Autodesk Inventor part; units mm, degrees
ref_plane "YZ Plane" through (0, 0, 0) normal (1, 0, 0) x (0, 1, 0)
ref_plane "XZ Plane" through (0, 0, 0) normal (0, 1, 0) x (-1, 0, 0)
ref_plane "XY Plane" through (0, 0, 0) normal (0, 0, 1) x (1, 0, 0)
sketch "Sketch1" plane through (0, 0, 0) normal (1, 0, 0) x (0, 1, 0)
  circle A0 centre (0, 0) radius 18.5
  dimension "d0" = 37
extrude "Extrusion1" add sketch "Sketch1" along normal blind 27
sketch "Sketch2" plane through (0, 0, 0) normal (-1, 0, 0) x (0, 0, 1)
  circle A0 centre (0, 0) radius 16
  dimension "d3" = 32
extrude "Extrusion2" add sketch "Sketch2" along normal blind 34
sketch "Sketch3" plane through (27, 0, 0) normal (1, 0, 0) x (0, 0, -1)
  circle A0 centre (0, 15.5) radius 1.5
  circle A1 centre (-13.4234, 7.75) radius 1.5
  circle A2 centre (-13.4234, -7.75) radius 1.5
  circle A3 centre (0, -15.5) radius 1.5
  circle A4 centre (13.4234, -7.75) radius 1.5
  circle A5 centre (13.4234, 7.75) radius 1.5
  point P0 (0, 0)
  dimension "d8" = 3
  dimension "d9" = 15.5
  dimension "d12" = 360
extrude "Extrusion3" cut sketch "Sketch3" against normal blind 3
sketch "Sketch4" plane through (27, 0, 0) normal (1, 0, 0) x (0, 0, -1)
  circle A0 centre (-7, 0) radius 6
  point P0 (0, 0)
  dimension "d16" = 12
  dimension "d17" = 7
extrude "Extrusion4" add sketch "Sketch4" along normal blind 6
sketch "Sketch5" plane through (33, 0, 7) normal (1, 0, 0) x (0, 0, -1)
  circle A0 centre (0, 0) radius 3
  point P0 (7, 0)
  dimension "d20" = 6
  dimension "d21" = 7
extrude "Extrusion5" add sketch "Sketch5" along normal blind 15.5
properties part number "SPG30_Motor"
Input: part model. Units: mm. Frame: model coordinates. A direction names the side the tool comes from. Round coordinates to 2 decimals unless told otherwise and drop trailing zeros. Loops run counter-clockwise (first coordinate to the right, second up) from the corner with the lowest first, then second, coordinate; pieces in that order, holes last.
1) Pull-direction query (Y, two-part tool) for faces 3 (the cylindrical face through (25.52, -8.32, -14.81)), 4 (the flat face through (0, -6, 15)), 5 (the cylindrical face through (40.64, 1.15, 4.23)); classes: released by +Y, released by -Y, zero draft, split by the parting line, or undercut.
Ans:
face 3: undercut
face 4: zero draft
face 5: split by the parting line
2) Set-up query: faces 1 (the cylindrical face through (-16.76, 15.62, -3.47)), 2 (the cylindrical face through (25.521, -8.663, 14.614)). Return all of +Z, -Z, +X, -X, +Y, -Y with unobstructed straight access to the full face (end or side cutting, diameter ignored); none if empty.
Ans:
face 1: -X
face 2: +X
3) Section query B-B on y = 0. Return the cut outline in (x, z).
Ans:
outline: (-34, -16) - (0, -16) - (0, -18.5) - (27, -18.5) - (27, 1) - (33, 1) - (33, 4) - (48.5, 4) - (48.5, 10) - (33, 10) - (33, 13) - (27, 13) - (27, 18.5) - (0, 18.5) - (0, 16) - (-34, 16) - close
4) Section query A-A on z = 6. Return the cut outline in (x, y), plus the area to 3 significant figures.
Ans:
outline: (-34, -14.83) - (0, -14.83) - (0, -17.5) - (27, -17.5) - (27, -5.92) - (33, -5.92) - (33, -2.83) - (48.5, -2.83) - (48.5, 2.83) - (33, 2.83) - (33, 5.92) - (27, 5.92) - (27, 17.5) - (0, 17.5) - (0, 14.83) - (-34, 14.83) - close
area: 2,110 mm2
5) Pin query (flat end, axial travel): pin 1 (4 mm diameter, centred on x = 17.5, y = -2.5, fed in from -Z); pin 2 (10 mm diameter, centred on x = -24.5, y = 2.5, fed in from +Z); pin 3 (1.5 mm diameter, centred on y = -8, z = -13.5, fed in from +X). Return the tip coordinate at first contact, or that it passes through.
Ans:
pin 1: stops at z = -18.49
pin 2: stops at z = 16
pin 3: stops at x = 24
6) Section query D-D on z = -6. Return the cut outline in (x, y).
Ans:
outline: (-34, -14.83) - (0, -14.83) - (0, -17.5) - (27, -17.5) - (27, 17.5) - (0, 17.5) - (0, 14.83) - (-34, 14.83) - close
7) Material intervals for line 1 (Z direction, x = 25, y = -7); line 2 (X direction, y = -14, z = 7.5); line 3 (X direction, y = -17, z = 4), sorted ascending.
Ans:
line 1: z = -17.12 to -14.72, -12.12 to 12.12, 14.72 to 17.12
line 2: x = -34 to 27
line 3: x = 0 to 27
8) Section query C-C on x = 35. Return the cut outline in (y, z).
Ans:
outline: circle Ø6 at (0, 7)
